Could you check a few things on this model? Use its own coordinates, in mm. Coordinates: 2 decimals unless noted, no trailing zeros. Loops run counter-clockwise (first coordinate to the right, second up) from the corner with the lowest first, then second, coordinate; pieces in that order, holes last.
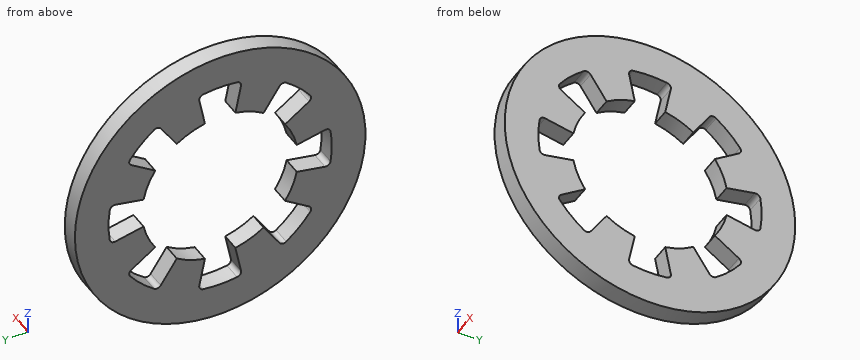
Autodesk Inventor part; units mm, degrees
ref_plane "Work Plane1" through (0, 0, 0) normal (0, 1, 0) x (1, 0, 0)
ref_plane "YZ Plane" through (0, 0, 0) normal (1, 0, 0) x (0, 1, 0)
ref_plane "XZ Plane" through (0, 0, 0) normal (0, 1, 0) x (-1, 0, 0)
sketch "Sketch1" plane through (0, 0, 0) normal (1, 0, 0) x (0, 1, 0)
  circle A0 centre (0, 0) radius 4
  circle A1 centre (0, 0) radius 2.15
  dimension "d0" = 8
  dimension "d1" = 4.3
extrude "Body" add sketch "Sketch1" along normal blind 0.5
sketch "Sketch2" plane through (0, 0, 0) normal (-1, 0, 0) x (0, 0, 1)
  circle A0 centre (0, 0) radius 2.15
  circle A1 centre (0, 0) radius 4
  arc A2 (0.5999, 3.0159) -> (-0.5999, 3.0159) centre (0, 0) ccw
  line L0 (-0.4194, 2.1087) -> (-0.5999, 3.0159)
  line L1 (0, 0) -> (0, 3.075) construction
  line L2 (0.4194, 2.1087) -> (0.5999, 3.0159)
  line L3 (-0.4194, 2.1087) -> (0, 0) construction
  line L4 (0.4194, 2.1087) -> (0, 0) construction
  dimension "d4" = 6.15
  dimension "d5" = 11.25
extrude "Cut" cut sketch "Sketch2" against normal blind 0.5 contours A0 L0 A2 L2
fillet "Fillet1" radius 0.129 2 edges at (0.25, 3.0159, 0.5999) (0.25, 3.0159, -0.5999)
pattern_circular "Cuts" count 8 over 360 about axis through (-10, 0, 0) along (1, 0, 0) of "Cut", "Fillet1"
ref_plane "Work Plane1" through (0, 0, 0) normal (0, 1, 0) x (1, 0, 0)
equation "\"d0\" = SD2"
equation "\"d1\" = SD1"
equation "\"d2\" = SD"
equation "\"d4\" = 0.5 * SD2 + 0.5 * SD1"
equation "\"d6\" = SD"
equation "\"d8\" = 0.03 * SD1"
equation "\"SD1\" = 4.3"
equation "\"SD2\" = 8"
equation "\"SD\" = 0.5"
equation "\"NND\" = 4"
properties part number "DIN 6797 - J 4.3" material "Steel, Mild"
(1) I need wall thicknesses on probe 1 along Z at (x, y) = (0.25, -2.25); probe 2 along Y at (x, z) = (0.45, 1.25); probe 3 along Y at (x, z) = (0.4, 1.75). Which ranges of each line are inside material? Lowest first, please.
Answers:
probe 1: z = -3.31 to -2.1, -1.5 to -0.45, 0.45 to 1.5, 2.1 to 3.31
probe 2: y = -3.8 to -1.87, 1.87 to 3.8
probe 3: y = -3.6 to -2.5, 2.5 to 3.6
(2) Imagine slicing it at D-D, the plane y = 2.25. Write out the boundary of the cut face in (x, z).
Answers:
outline: (0, -3.31) - (0.5, -3.31) - (0.5, -2.1) - (0, -2.1) - close; (0, -1.5) - (0.5, -1.5) - (0.5, -0.45) - (0, -0.45) - close; (0, 0.45) - (0.5, 0.45) - (0.5, 1.5) - (0, 1.5) - close; (0, 2.1) - (0.5, 2.1) - (0.5, 3.31) - (0, 3.31) - close
(3) Imagine slicing it at A-A, the plane y = 0. Write out the boundary of the cut face in (x, z), and give its area (3 significant figures).
Answers:
outline: (0, -4) - (0.5, -4) - (0.5, -3.07) - (0, -3.07) - close; (0, 3.07) - (0.5, 3.07) - (0.5, 4) - (0, 4) - close
area: 0.925 mm2
(4) Imagine slicing it at C-C, the plane y = -2. Write out the boundary of the cut face in (x, z).
Answers:
outline: (0, -3.46) - (0.5, -3.46) - (0.5, -2.34) - (0, -2.34) - close; (0, -1.34) - (0.5, -1.34) - (0.5, -0.79) - (0, -0.79) - close; (0, 0.79) - (0.5, 0.79) - (0.5, 1.34) - (0, 1.34) - close; (0, 2.34) - (0.5, 2.34) - (0.5, 3.46) - (0, 3.46) - close
